Input: part model. Units: mm. Frame: model coordinates. Face numbers are marked on the shaded views. A direction names the side the tool comes from. Coordinates: 2 decimals unless noted, no trailing zeros. Write each loop counter-clockwise with the first axis right and the second up, starting at its lowest first coordinate (ties: lowest second). Pieces come first, ordered by that corner, then holes. Notation, with made-up numbers: (22, 40.5) - (55, 40.5) arc R3 cw to (55, 44.5) - close; hole circle Ø3 at (78, -19.75). An arc over 180 degrees is marked (long way). Put each result on its own line as item: value. Start each with the question number.
1. Pull-direction query (X, two-part tool) for the marked faces 3, 4 and 5; classes: released by +X, released by -X, zero draft, split by the parting line, or undercut.
2. Line query: line 1 (Z direction, x = -0.7, y = -0.85); line 2 (Y direction, x = 0.5, z = 4.1); line 3 (Y direction, x = -2, z = 5.6). Output: solid intervals per line, ascending.
3. Cut plane A-A, the plane x = 0. Return loops of the section in (y, z).
4. Access query for the marked faces 1 and 2. Directions: +Z, -Z, +X, -X, +Y, -Y. A direction counts if a zero-diameter tool reaches every point of the face in a straight line with its end or side. Return the directions, or none.
5. Cut plane B-B, the plane z = 2.35. Return loops of the section in (x, y), and give its area (3 significant figures).
6. Pin query (flat end, axial travel): pin 1 (3 mm diameter, centred on y = 2, z = 1, fed in from +X); pin 2 (0.9 mm diameter, centred on x = 0.5, y = 0, fed in from +Z). Return the tip coordinate at first contact, or that it passes through.
Autodesk Inventor part; units mm, degrees
ref_plane "YZ Plane" through (0, 0, 0) normal (1, 0, 0) x (0, 1, 0)
ref_plane "XZ Plane" through (0, 0, 0) normal (0, 1, 0) x (-1, 0, 0)
ref_plane "XY Plane" through (0, 0, 0) normal (0, 0, 1) x (1, 0, 0)
sketch "Sketch1" plane through (0, 0, 0) normal (0, 0, 1) x (1, 0, 0)
  circle A0 centre (0, 0) radius 2.5
  dimension "Dia" = 5
extrude "Extrusion1" add sketch "Sketch1" along normal blind 6
chamfer "Chamfer1" distance 0.5 angle 45 1 edges at (-2.5, 0, 0)
thread "Thread1"
sketch "Sketch2" plane through (0, 0, 6) normal (0, 0, 1) x (1, 0, 0)
  line L0 (0.866, 1.5) -> (1.7321, 0)
  line L1 (1.7321, 0) -> (0.866, -1.5)
  line L2 (0.866, -1.5) -> (-0.866, -1.5)
  line L3 (-0.866, -1.5) -> (-1.7321, 0)
  line L4 (-1.7321, 0) -> (-0.866, 1.5)
  line L5 (-0.866, 1.5) -> (0.866, 1.5)
  point P0 (0, 0)
  dimension "d8" = 3
extrude "Extrusion2" cut sketch "Sketch2" against normal blind 2
equation "\"d3\" = 0.1 * Dia"
properties part number "24-506-5F" material "Steel, High Strength Low Alloy"
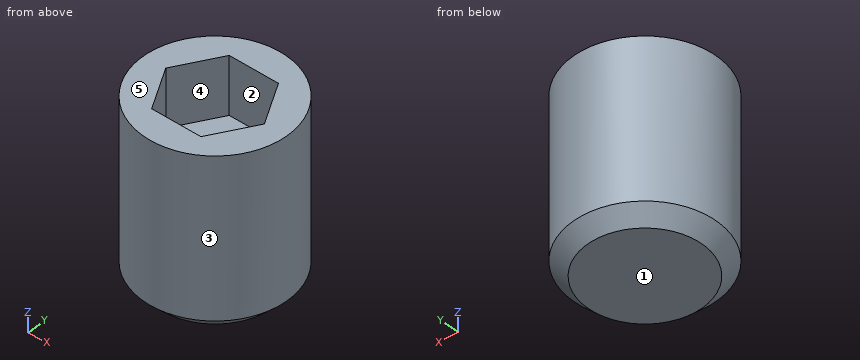
Report:
1. face 3: split by the parting line
1. face 4: undercut
1. face 5: zero draft
2. line 1: z = 0 to 4
2. line 2: y = -2.45 to -1.5, 1.5 to 2.45
2. line 3: y = -1.5 to 1.5
3. outline: (-2.5, 0.5) - (-2, 0) - (2, 0) - (2.5, 0.5) - (2.5, 6) - (1.5, 6) - (1.5, 4) - (-1.5, 4) - (-1.5, 6) - (-2.5, 6) - close
4. face 1: -Z, +X, -X, +Y, -Y
4. face 2: +Z
5. outline: circle Ø5 at (0, 0)
5. area: 19.6 mm^2
6. pin 1: stops at x = 2.45
6. pin 2: stops at z = 4
